Can you work these out from the model? Positions are in its coordinate system, mm. Face numbers are marked on the shaded views. A direction names the side the tool comes from. Coordinates: 2 decimals unless noted, no trailing zeros. Order: outer loops, then holes, each group sorted by start corner. A loop starts at its lowest first (then second) coordinate and runs counter-clockwise, first axis right, second up. Notation, with made-up numbers: (20.25, 5) - (31.25, 5) arc R23 ccw to (31.25, 41) - close; hole circle Ø3 at (86.5, -12.5). An arc over 180 degrees is marked (long way). Return JSON: item names as keys, results as strings. Group by question number.
1) Imagine slicing it at B-B (y = -4.5). Write out the boundary of the cut face in (x, z), and give its area (3 significant figures).
2) Imagine slicing it at D-D (z = 2). Write out the boundary of the cut face in (x, y), and give its area (3 significant figures).
3) Imagine slicing it at A-A (z = 7.25). Write out the boundary of the cut face in (x, y), and give its area (3 significant figures).
4) If we mould it in two halves opening along Y, with no side actions, what happens to the marked faces 1, 2 and 3? For each: pulls with the +Y half, pulls with the -Y half, needs draft (parallel to the pull), parting line crosses it, or undercut.
5) Imagine slicing it at C-C (x = 1.2). Write out the boundary of the cut face in (y, z), and give its area (3 significant figures).
6) If I drill on line 1 along Y through (x, z) = (0.35, 4.5); line 2 along Y through (x, z) = (0.75, 5); line 3 along Y through (x, z) = (0.15, 1.25), over which ranges is the centre line in solid material (lowest first)?
7) Which directions (+Z, -Z, +X, -X, +Y, -Y) give clear straight access to the entire face, cutting with the end or side of a thin tool? Please do the marked faces 4 and 5.
8) For pin 1 Ø1.5 at (x, z) = (1, 3) entering from +Y; pin 2 Ø1.3 at (y, z) = (-1.39, 4.86) entering from +X; pin 3 Ø0.6 at (y, z) = (-9.5, 7.5) entering from +X; pin 4 Ø3 at (x, y) = (0, -1.5) entering from +Z, each with a flat end and sliding along its axis, tell me the tip position at first contact or that it passes through.
```python
from build123d import *

# Parameters (mm, degrees)
SKETCH2_W           = 5.7404
SKETCH2_H           = 12.8143
OG_BOX_DEPTH        = 6.0452
SKETCH4_W           = 0.508
SKETCH4_H           = 0.762
PINS_DEPTH          = 3.175
CLICKER_DEPTH       = 3.5814
SKETCH8_W           = 5.7404
SKETCH8_H           = 2.54
BOSS_EXTRUDE3_DEPTH = 0.381
SKETCH9_R           = 1.0541
CUT_EXTRUDE1_DEPTH  = 8.89


with BuildPart() as part:
    # Sketch2 → OG box (new body)
    with BuildSketch(Plane.XY):
        with Locations((0.019740217, -4.616841123)):
            Rectangle(SKETCH2_W, SKETCH2_H)
    extrude(amount=OG_BOX_DEPTH)

    # Sketch4 → Pins (add)
    with BuildSketch(Plane.XY.offset(6.0452)):
        with Locations((0, -4.616841123)):
            Rectangle(SKETCH4_W, SKETCH4_H)
        with Locations((0, 0.513958877)):
            Rectangle(SKETCH4_W, SKETCH4_H)
        with Locations((0, -9.747641123)):
            Rectangle(SKETCH4_W, SKETCH4_H)
    extrude(amount=PINS_DEPTH)

    # Sketch6 → Clicker (add)
    with BuildSketch(Plane.ZY.offset(1.7907)):
        Polygon((0, -10.56854726), (-3.5867143, 2.81725274), (-3.292300108, 2.896140785), (-2.938516926, 1.575803975), (0, -9.390890493), align=None)
    extrude(amount=-CLICKER_DEPTH)

    # Sketch8 → Boss-Extrude3 (add)
    with BuildSketch(Plane.XY.offset(6.0452)):
        with Locations((0.019740217, -1.391041123)):
            Rectangle(SKETCH8_W, SKETCH8_H)
        with Locations((0.019740217, -7.842641123)):
            Rectangle(SKETCH8_W, SKETCH8_H)
    extrude(amount=BOSS_EXTRUDE3_DEPTH)

    # Sketch9 → Cut-Extrude1 (cut)
    with BuildSketch(Plane(origin=(2.889940217, 0, 0), x_dir=(0, 0, -1), z_dir=(1, 0, 0))):
        with Locations(Location((-4.8641, -1.391041123, 0), (0, 0, 90))):
            Circle(SKETCH9_R)
        with Locations(Location((-4.8641, -7.842641123, 0), (0, 0, 90))):
            Circle(SKETCH9_R)
    extrude(amount=-CUT_EXTRUDE1_DEPTH, mode=Mode.SUBTRACT)


solid = part.part
```
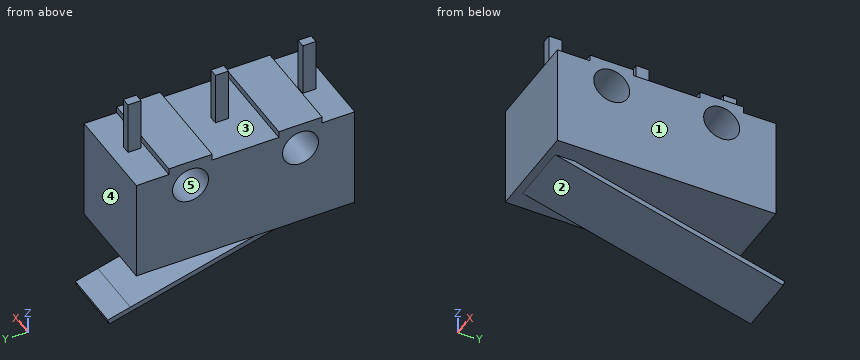
Calculated:
{
 "1": {"outline": "(-2.85, 0) - (2.89, 0) - (2.89, 6.05) - (0.25, 6.05) - (0.25, 9.22) - (-0.25, 9.22) - (-0.25, 6.05) - (-2.85, 6.05) - close; (-1.79, -1.63) - (1.79, -1.63) - (1.79, -1.31) - (-1.79, -1.31) - close", "area": "37.4 mm2"},
 "2": {"outline": "(-2.85, -11.02) - (2.89, -11.02) - (2.89, 1.79) - (-2.85, 1.79) - close", "area": "73.6 mm2"},
 "3": {"outline": "(-0.25, -10.13) - (0.25, -10.13) - (0.25, -9.37) - (-0.25, -9.37) - close; (-0.25, -5) - (0.25, -5) - (0.25, -4.24) - (-0.25, -4.24) - close; (-0.25, 0.13) - (0.25, 0.13) - (0.25, 0.89) - (-0.25, 0.89) - close", "area": "1.16 mm2"},
 "4": {"face 1": "needs draft", "face 2": "pulls with the -Y half", "face 3": "undercut"},
 "5": {"outline": "(-11.02, 0) - (-10.57, 0) - (2.82, -3.59) - (2.9, -3.29) - (-9.39, 0) - (1.79, 0) - (1.79, 6.05) - (-0.12, 6.05) - (-0.12, 6.43) - (-2.66, 6.43) - (-2.66, 6.05) - (-6.57, 6.05) - (-6.57, 6.43) - (-9.11, 6.43) - (-9.11, 6.05) - (-11.02, 6.05) - close; hole circle Ø2.11 at (-7.84, 4.86); hole circle Ø2.11 at (-1.39, 4.86)", "area": "76.5 mm2"},
 "6": {"line 1": "-11.02 to -8.83, -6.85 to -2.38, -0.4 to 1.79", "line 2": "-11.02 to -8.89, -6.8 to -2.44, -0.35 to 1.79", "line 3": "-11.02 to 1.79"},
 "7": {"face 4": "+Z, +X, -X, +Y", "face 5": "+X, -X"},
 "8": {"pin 1": "y = 1.79", "pin 2": "through", "pin 3": "x = 0.25", "pin 4": "z = 6.43"}
}
